```python
from build123d import *

# Parameters (mm, degrees)
PAD_DEPTH   = 160
FILLET_R    = 10
FILLET001_R = 7.5


with BuildPart() as part:
    # Sketch → Pad (new body)
    with BuildSketch(Plane.XY):
        Polygon((0, 0), (70, 0), (70, 8), (4, 8), (4, 18), (8, 18), (8, 70), (0, 70), (-4, 26), (-4, 0), align=None)
    extrude(amount=PAD_DEPTH)

    # Fillet
    fillet_edges = [part.edges().sort_by_distance(p)[0] for p in [
        (-4, 0, 80),
    ]]
    fillet(fillet_edges, radius=FILLET_R)

    # Fillet001
    fillet001_edges = [part.edges().sort_by_distance(p)[0] for p in [
        (0, 70, 80),
        (70, 0, 80),
    ]]
    fillet(fillet001_edges, radius=FILLET001_R)


solid = part.part
```
Work out the finished part from the listing and answer in its coordinate system (mm). A direction names the side the tool comes from. Give positions to 0.01 mm unless a question says otherwise; leave off trailing zeros. Loops run counter-clockwise (first coordinate to the right, second up) from the corner with the lowest first, then second, coordinate; pieces in that order, holes last. Notation, with made-up numbers: (-1.5, 79) -> (36.5, 79) arc R26 cw to (36.5, 100) -> close; hole circle Ø5 at (52, 57). An arc over 180 degrees is marked (long way). Use CSV: the item, a comma, the result in double quotes.
1. The mould has two halves that part along Y. Classify faces 1 (the flat face through (4, 13, 79)), 2 (the flat face through (6, 18, 79)), 3 (the cylindrical face through (67.745, 2.139, 81.12)), 4 (the flat face through (5, 22, 0)): +Y half, -Y half, draft (parallel to the pull), parting line (faces both ways), or undercut.
Found:
face 1,"undercut"
face 2,"undercut"
face 3,"-Y half"
face 4,"draft"
2. A tool of negligible diameter and unlimited length cuts with its end or side. For faces 5 (the flat face through (-4, 18, 79)), 6 (the flat face through (8, 44, 79)), from which of +Z, -Z, +X, -X, +Y, -Y can it reach the whole face along a straight path? Write none if from no direction.
Found:
face 5,"+Z, -Z, -X, +Y, -Y"
face 6,"+Z, -Z, +X, +Y"
3. The part is cut by section C-C (x = 34.5). Write down the section's boundary in (y, z), then the cut area to 3 significant figures.
Found:
outline,"(0, 0) -> (8, 0) -> (8, 160) -> (0, 160) -> close"
area,"1,280 mm^2"
4. The part is cut by section A-A (z = 69.5). Write down the section's boundary in (x, y).
Found:
outline,"(-4, 10) arc R10 ccw to (6, 0) -> (62.5, 0) arc R7.5 ccw to (70, 7.5) -> (70, 8) -> (4, 8) -> (4, 18) -> (8, 18) -> (8, 70) -> (6.85, 70) arc R7.5 ccw to (-0.62, 63.18) -> (-4, 26) -> close"
5. Straight lines are drawn through the part: line 1 (Y direction, x = 7, z = 150.5); line 2 (Y direction, x = 9, z = 44.5); line 3 (X direction, y = 14.5, z = 111). For each, find the intervals that lie inside material, in ascending order.
Found:
line 1,"0 to 8, 18 to 70"
line 2,"0 to 8"
line 3,"-4 to 4"
6. Flat-ended cylindrical pins translate along their axes: pin 1 Ø3 at (x, z) = (32, 21) entering from +Y; pin 2 Ø3 at (y, z) = (11, 118) entering from +X; pin 3 Ø2 at (y, z) = (29.5, 64.5) entering from +X. Find the tip coordinate at first contact, or state that the pin passes through.
Found:
pin 1,"y = 8"
pin 2,"x = 4"
pin 3,"x = 8"
7. The part is cut by section B-B (y = 13.5). Write down the section's boundary in (x, z).
Found:
outline,"(-4, 0) -> (4, 0) -> (4, 160) -> (-4, 160) -> close"
